Design review of the part built by this model. Coordinates are the model's own, in mm. Face numbers are marked on the shaded views. A direction names the side the tool comes from. Coordinates: 2 decimals unless noted, no trailing zeros. Write each loop counter-clockwise with the first axis right and the second up, starting at its lowest first coordinate (ties: lowest second). Pieces come first, ordered by that corner, then holes.
Q1. Take a section at D-D, the plane x = -9. Write out the cut boundary in (y, z).
Q2. The part is to be moulded in two halves that separate along X. For the marked faces 3, 4, 5 and 6, say which applies: released by +X, released by -X, zero draft, split by the parting line, or undercut.
Q3. Take a section at C-C, the plane y = 4.5. Write out the cut boundary in (x, z), plus the area to 3 significant figures.
Q4. For pin 1 Ø9 at (x, z) = (0, 0) entering from +Y; pin 2 Ø2 at (x, y) = (2.5, 2.5) entering from -Z; pin 3 Ø4 at (x, y) = (5.5, 1.5) entering from +Z; pin 4 Ø3 at (x, y) = (7, 5) entering from -Z, all flat-tipped, find the tip position at first contact; note any pin that passes through.
Q5. Take a section at A-A, the plane z = 0. Write out the cut boundary in (x, y) (3 decimals).
Q6. For the marked faces 1 and 2, list the 3-axis set-ups (+Z, -Z, +X, -X, +Y, -Y) from which the entire face can be reached by the end or side of a thin tool; tool diameter is ignored.
Q7. Take a section at B-B, the plane x = 1.5. Write out the cut boundary in (y, z), plus the area to 3 significant figures.
Q8. For L1, parallel to X at y = 3.5, z = 0; L2, parallel to Y at x = -6.5, z = -11.25; L3, parallel to Z at x = -3.75, y = 4.25, list the stretches that pass through material, from the lowest coordinate up.
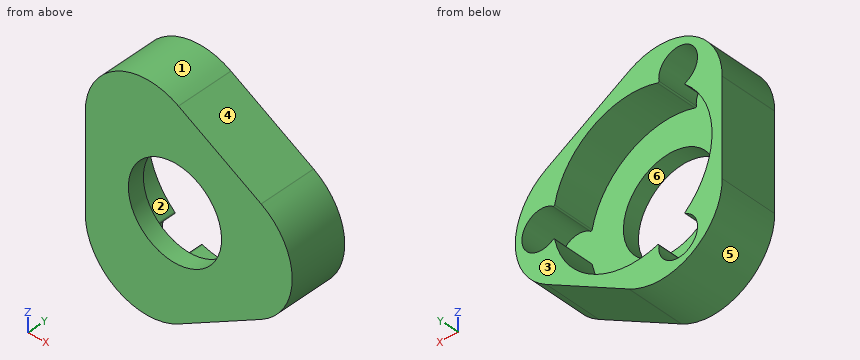
from build123d import *

# Parameters (mm, degrees)
BOSS_EXTRUDE15_DEPTH = 7
CUT_EXTRUDE1_DEPTH   = 5
SKETCH9_R            = 5.715
CUT_EXTRUDE2_DEPTH   = 5


with BuildPart() as part:
    # Sketch7 → Boss-Extrude15 (new body)
    with BuildSketch(Plane(origin=(0, 0, 0), x_dir=(1, 0, 0), z_dir=(0, 1, 0))):
        with BuildLine():
            Line((10.57, 6.599113577), (0.43, 12.453445306))
            ThreePointArc((0.43, 12.453445306), (-7.19, 12.453445306), (-11, 5.85433173))
            Line((-11, 5.85433173), (-11, -5.85433173))
            ThreePointArc((-11, -5.85433173), (-7.19, -12.453445306), (0.43, -12.453445306))
            Line((0.43, -12.453445306), (10.57, -6.599113577))
            ThreePointArc((10.57, -6.599113577), (14.38, 0), (10.57, 6.599113577))
        make_face()
    extrude(amount=BOSS_EXTRUDE15_DEPTH)

    # Sketch8 → Cut-Extrude1 (cut)
    with BuildSketch(Plane(origin=(0, 7, 0), x_dir=(1, 0, 0), z_dir=(0, 1, 0))):
        with BuildLine():
            ThreePointArc((-6.51776578, -7.494688754), (-6.784903319, -11.751797273), (-3.231707964, -9.391895118))
            ThreePointArc((-3.231707964, -9.391895118), (-3.186361585, -9.277920027), (-3.065770585, -9.255460589))
            ThreePointArc((-3.065770585, -9.255460589), (4.875, -8.443747687), (9.548349287, -1.972695086))
            ThreePointArc((9.548349287, -1.972695086), (9.62809523, -1.879489935), (9.749473744, -1.897206364))
            ThreePointArc((9.749473744, -1.897206364), (13.569806638, 0), (9.749473744, 1.897206364))
            ThreePointArc((9.749473744, 1.897206364), (9.62809523, 1.879489935), (9.548349287, 1.972695086))
            ThreePointArc((9.548349287, 1.972695086), (4.875, 8.443747687), (-3.065770585, 9.255460589))
            ThreePointArc((-3.065770585, 9.255460589), (-3.186361585, 9.277920027), (-3.231707964, 9.391895118))
            ThreePointArc((-3.231707964, 9.391895118), (-6.784903319, 11.751797273), (-6.51776578, 7.494688754))
            ThreePointArc((-6.51776578, 7.494688754), (-6.441733645, 7.398430092), (-6.482578701, 7.282765504))
            ThreePointArc((-6.482578701, 7.282765504), (-9.75, 0), (-6.482578701, -7.282765504))
            ThreePointArc((-6.482578701, -7.282765504), (-6.441733645, -7.398430092), (-6.51776578, -7.494688754))
        make_face()
    extrude(amount=-CUT_EXTRUDE1_DEPTH, mode=Mode.SUBTRACT)

    # Sketch9 → Cut-Extrude2 (cut)
    with BuildSketch(Plane(origin=(0, 2, 0), x_dir=(1, 0, 0), z_dir=(0, 1, 0))):
        with Locations(Location((0, 0, 0), (0, 0, 270))):
            Circle(SKETCH9_R)
    extrude(amount=-CUT_EXTRUDE2_DEPTH, mode=Mode.SUBTRACT)


solid = part.part
Responses:
1. outline: (0, -11) - (7, -11) - (7, -3.75) - (2, -3.75) - (2, 3.75) - (7, 3.75) - (7, 11) - (0, 11) - close
2. face 3: zero draft
2. face 4: released by +X
2. face 5: split by the parting line
2. face 6: undercut
3. outline: (-11, -5.85) arc R7.62 ccw to (0.43, -12.45) - (10.57, -6.6) arc R7.62 ccw to (10.57, 6.6) - (0.43, 12.45) arc R7.62 ccw to (-11, 5.85) - close; hole (-6.52, -7.49) arc R2.38 ccw (long way) to (-3.23, -9.39) arc R0.13 cw to (-3.07, -9.26) arc R9.75 ccw to (9.55, -1.97) arc R0.13 cw to (9.75, -1.9) arc R2.38 ccw (long way) to (9.75, 1.9) arc R0.13 cw to (9.55, 1.97) arc R9.75 ccw to (-3.07, 9.26) arc R0.13 cw to (-3.23, 9.39) arc R2.38 ccw (long way) to (-6.52, 7.49) arc R0.13 cw to (-6.48, 7.28) arc R9.75 ccw to (-6.48, -7.28) arc R0.13 cw to start
3. area: 164 mm2
4. pin 1: passes through
4. pin 2: stops at z = -11.84
4. pin 3: stops at z = 10.68
4. pin 4: stops at z = -9.53
5. outline: (-11, 0) - (-5.715, 0) - (-5.715, 2) - (-9.75, 2) - (-9.75, 7) - (-11, 7) - close; (5.715, 0) - (14.38, 0) - (14.38, 7) - (13.57, 7) - (13.57, 2) - (5.715, 2) - close
6. face 1: +Z, +Y, -Y
6. face 2: +Y
7. outline: (0, -11.84) - (7, -11.84) - (7, -9.63) - (2, -9.63) - (2, -5.51) - (0, -5.51) - close; (0, 5.51) - (2, 5.51) - (2, 9.63) - (7, 9.63) - (7, 11.84) - (0, 11.84) - close
7. area: 47.3 mm2
8. L1: x = -11 to -9.75, 13.57 to 14.38
8. L2: y = 0 to 2
8. L3: z = -13.47 to -11.2, 11.2 to 13.47
